Could you check a few things on this model? Use its own coordinates, in mm. Round coordinates to 2 decimals unless told otherwise and drop trailing zeros. Order: outer loops, then holes, each group sorted by start corner. A loop starts at its lowest first (then second) coordinate and runs counter-clockwise, first axis right, second up. Notation, with made-up numbers: (81.25, 80) - (96.25, 80) arc R24 cw to (96.25, 91) - close; hole circle Ø10 at (34.5, 6.25). An arc over 180 degrees is marked (long way). Use one line per item in the form item = value.
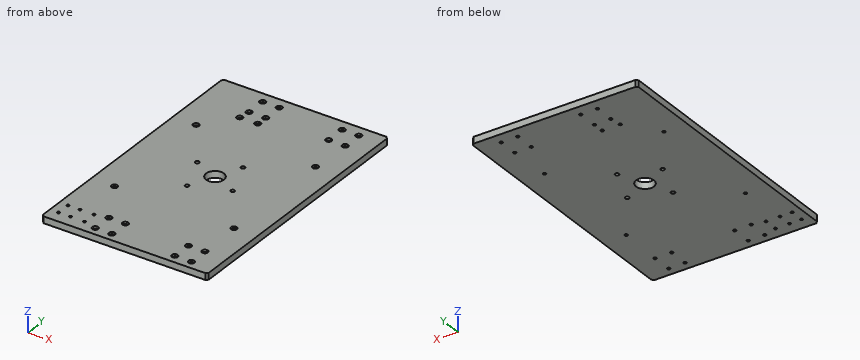
from build123d import *

# Parameters (mm, degrees)
ESQUISSE1_W                                  = 250
ESQUISSE1_H                                  = 400
BOSS_EXTRU_1_DEPTH                           = 10
ESQUISSE2_R                                  = 13.5
ENL_V_MAT_EXTRU_1_DEPTH                      = 237.061432682
CHANFREIN1_SIZE                              = 3
TROU_TARAUD_M51_D                            = 4.2
TROUS_DE_CENTRAGE_4_0MM2_D                   = 4
TROUS_DE_CENTRAGE_6_0MM2_D                   = 6
D_GAGEMENT_M41_D                             = 4.5
R_P_TITION_LIN_AIRE1_COUNT                   = 2
R_P_TITION_LIN_AIRE1_PITCH                   = 120
R_P_TITION_LIN_AIRE1_COUNT_DIR2              = 2
R_P_TITION_LIN_AIRE1_PITCH_DIR2              = 340
R_P_TITION_LIN_AIRE2_COUNT                   = 2
R_P_TITION_LIN_AIRE2_PITCH                   = 30
R_P_TITION_LIN_AIRE2_COUNT_DIR2              = 2
R_P_TITION_LIN_AIRE2_PITCH_DIR2              = 25
R_P_TITION_LIN_AIRE3_COUNT                   = 2
R_P_TITION_LIN_AIRE3_PITCH                   = 120
R_P_TITION_LIN_AIRE3_COUNT_DIR2              = 2
R_P_TITION_LIN_AIRE3_PITCH_DIR2              = 340
D_GAGEMENT_M42_D                             = 4.5
CHAMBRAGE_POUR_VIS_T_TE_RONDE_BOMB_2_A_COUNT = 2
CHAMBRAGE_POUR_VIS_T_TE_RONDE_BOMB_2_A_PITCH = 180
CHAMBRAGE_POUR_VIS_T_TE_RONDE_BOMB_3_COUNT   = 2
CHAMBRAGE_POUR_VIS_T_TE_RONDE_BOMB_3_PITCH   = 180
CHAMBRAGE_POUR_VIS_T_TE_RONDE_BOMB_4_COUNT   = 2
CHAMBRAGE_POUR_VIS_T_TE_RONDE_BOMB_4_PITCH   = 254.558441227
D_GAGEMENT_M43_D                             = 4.5
CHAMBRAGE_POUR_VIS_T_TE_RONDE_BOMB_5_A_COUNT = 2
CHAMBRAGE_POUR_VIS_T_TE_RONDE_BOMB_5_A_PITCH = 26.858717456


with BuildPart() as part:
    # Esquisse1 → Boss.-Extru.1 (new body)
    with BuildSketch(Plane.XY):
        Rectangle(ESQUISSE1_W, ESQUISSE1_H)
    extrude(amount=BOSS_EXTRU_1_DEPTH)

    # Esquisse2 → Enlèv. mat.-Extru.1 (cut, through all)
    with BuildSketch(Plane(origin=(0, 0, 0), x_dir=(-1, 0, 0), z_dir=(0, 0, -1))):
        Circle(ESQUISSE2_R)
    extrude(amount=-ENL_V_MAT_EXTRU_1_DEPTH, mode=Mode.SUBTRACT)

    # Chanfrein1
    chanfrein1_edges = [part.edges().sort_by_distance(p)[0] for p in [
        (125, -200, 5),
        (-125, -200, 5),
        (-125, 200, 5),
        (125, 200, 5),
    ]]
    chamfer(chanfrein1_edges, length=CHANFREIN1_SIZE)

    # Trou taraudé M51 (through all)
    with Locations(Plane.XY.offset(10)):
        with Locations((-72.698486264, -161.07971462), (-72.698486264, -181.838730229), (-111.937151978, -181.838730229), (-111.937151978, -161.07971462)):
            Hole(TROU_TARAUD_M51_D / 2)

    # Trous de centrage Ø4.0mm2 (through all)
    with Locations(Plane.XY.offset(10)):
        with Locations((-93.86308218, -161.07971462), (-93.86308218, -181.838730229)):
            Hole(TROUS_DE_CENTRAGE_4_0MM2_D / 2)

    # Trous de centrage Ø6.0mm2 (through all)
    with Locations(Plane.XY.offset(10)):
        with Locations((16.357059687, 37.86831259), (37.86831259, -16.357059687), (-16.357059687, -37.86831259), (-37.86831259, 16.357059687)):
            Hole(TROUS_DE_CENTRAGE_6_0MM2_D / 2)

    # Dégagement M41 (through all)
    with Locations(Plane(origin=(0, 0, 0), x_dir=(-1, 0, 0), z_dir=(0, 0, -1))):
        with Locations((28, -187), (28, -157), (53, -157), (53, -187)):
            d_gagement_m41 = Hole(D_GAGEMENT_M41_D / 2)

    # Répétition linéaire1: D_gagement M41 2 × 2
    with Locations(*[(i * R_P_TITION_LIN_AIRE1_PITCH, j * R_P_TITION_LIN_AIRE1_PITCH_DIR2, 0) for i in range(R_P_TITION_LIN_AIRE1_COUNT) for j in range(R_P_TITION_LIN_AIRE1_COUNT_DIR2) if (i, j) != (0, 0)]):
        add(d_gagement_m41, mode=Mode.SUBTRACT)

    # Esquisse29 → Chambrage pour vis _ t_te ronde bomb_e M (revolve, cut)
    with BuildSketch(Plane(origin=(92, -157, 10), x_dir=(0, -1, 0), z_dir=(1, 0, 0))):
        Polygon((0, 0), (0, 10), (2.25, 10), (2.25, 3.125), (2.275, 3.1), (4.5, 3.1), (4.5, 0), align=None)
    chambrage_pour_vis_t_te_ronde_bomb_e_m = revolve(axis=Axis((92, -157, 16.35), (0, 0, -1)), mode=Mode.SUBTRACT)

    # Répétition linéaire2: Chambrage pour vis _ t_te ronde bomb_e M 2 × 2
    with Locations(*[(-j * R_P_TITION_LIN_AIRE2_PITCH_DIR2, -i * R_P_TITION_LIN_AIRE2_PITCH, 0) for i in range(R_P_TITION_LIN_AIRE2_COUNT) for j in range(R_P_TITION_LIN_AIRE2_COUNT_DIR2) if (i, j) != (0, 0)]):
        add(chambrage_pour_vis_t_te_ronde_bomb_e_m, mode=Mode.SUBTRACT)

    # Répétition linéaire3: Chambrage pour vis _ t_te ronde bomb_e M 2 × 2
    with Locations(*[(-i * R_P_TITION_LIN_AIRE3_PITCH, j * R_P_TITION_LIN_AIRE3_PITCH_DIR2, 0) for i in range(R_P_TITION_LIN_AIRE3_COUNT) for j in range(R_P_TITION_LIN_AIRE3_COUNT_DIR2) if (i, j) != (0, 0)]):
        add(chambrage_pour_vis_t_te_ronde_bomb_e_m, mode=Mode.SUBTRACT)

    # Répétition linéaire3 copy 1 sketch → Répétition linéaire3 copy 1 (revolve, cut)
    with BuildSketch(Plane(origin=(67, 183, 10), x_dir=(0, -1, 0), z_dir=(1, 0, 0))):
        Polygon((0, 0), (0, 10), (2.25, 10), (2.25, 3.125), (2.275, 3.1), (4.5, 3.1), (4.5, 0), align=None)
    revolve(axis=Axis((67, 183, 16.35), (0, 0, -1)), mode=Mode.SUBTRACT)

    # Répétition linéaire3 copy 2 sketch → Répétition linéaire3 copy 2 (revolve, cut)
    with BuildSketch(Plane(origin=(-53, -157, 10), x_dir=(0, -1, 0), z_dir=(1, 0, 0))):
        Polygon((0, 0), (0, 10), (2.25, 10), (2.25, 3.125), (2.275, 3.1), (4.5, 3.1), (4.5, 0), align=None)
    revolve(axis=Axis((-53, -157, 16.35), (0, 0, -1)), mode=Mode.SUBTRACT)

    # Répétition linéaire3 copy 3 sketch → Répétition linéaire3 copy 3 (revolve, cut)
    with BuildSketch(Plane(origin=(-53, 183, 10), x_dir=(0, -1, 0), z_dir=(1, 0, 0))):
        Polygon((0, 0), (0, 10), (2.25, 10), (2.25, 3.125), (2.275, 3.1), (4.5, 3.1), (4.5, 0), align=None)
    revolve(axis=Axis((-53, 183, 16.35), (0, 0, -1)), mode=Mode.SUBTRACT)

    # Répétition linéaire3 copy 4 sketch → Répétition linéaire3 copy 4 (revolve, cut)
    with BuildSketch(Plane(origin=(92, 153, 10), x_dir=(0, -1, 0), z_dir=(1, 0, 0))):
        Polygon((0, 0), (0, 10), (2.25, 10), (2.25, 3.125), (2.275, 3.1), (4.5, 3.1), (4.5, 0), align=None)
    revolve(axis=Axis((92, 153, 16.35), (0, 0, -1)), mode=Mode.SUBTRACT)

    # Répétition linéaire3 copy 5 sketch → Répétition linéaire3 copy 5 (revolve, cut)
    with BuildSketch(Plane(origin=(-28, -187, 10), x_dir=(0, -1, 0), z_dir=(1, 0, 0))):
        Polygon((0, 0), (0, 10), (2.25, 10), (2.25, 3.125), (2.275, 3.1), (4.5, 3.1), (4.5, 0), align=None)
    revolve(axis=Axis((-28, -187, 16.35), (0, 0, -1)), mode=Mode.SUBTRACT)

    # Répétition linéaire3 copy 6 sketch → Répétition linéaire3 copy 6 (revolve, cut)
    with BuildSketch(Plane(origin=(-28, 153, 10), x_dir=(0, -1, 0), z_dir=(1, 0, 0))):
        Polygon((0, 0), (0, 10), (2.25, 10), (2.25, 3.125), (2.275, 3.1), (4.5, 3.1), (4.5, 0), align=None)
    revolve(axis=Axis((-28, 153, 16.35), (0, 0, -1)), mode=Mode.SUBTRACT)

    # Répétition linéaire3 copy 7 sketch → Répétition linéaire3 copy 7 (revolve, cut)
    with BuildSketch(Plane(origin=(67, 153, 10), x_dir=(0, -1, 0), z_dir=(1, 0, 0))):
        Polygon((0, 0), (0, 10), (2.25, 10), (2.25, 3.125), (2.275, 3.1), (4.5, 3.1), (4.5, 0), align=None)
    revolve(axis=Axis((67, 153, 16.35), (0, 0, -1)), mode=Mode.SUBTRACT)

    # Répétition linéaire3 copy 8 sketch → Répétition linéaire3 copy 8 (revolve, cut)
    with BuildSketch(Plane(origin=(-53, -187, 10), x_dir=(0, -1, 0), z_dir=(1, 0, 0))):
        Polygon((0, 0), (0, 10), (2.25, 10), (2.25, 3.125), (2.275, 3.1), (4.5, 3.1), (4.5, 0), align=None)
    revolve(axis=Axis((-53, -187, 16.35), (0, 0, -1)), mode=Mode.SUBTRACT)

    # Répétition linéaire3 copy 9 sketch → Répétition linéaire3 copy 9 (revolve, cut)
    with BuildSketch(Plane(origin=(-53, 153, 10), x_dir=(0, -1, 0), z_dir=(1, 0, 0))):
        Polygon((0, 0), (0, 10), (2.25, 10), (2.25, 3.125), (2.275, 3.1), (4.5, 3.1), (4.5, 0), align=None)
    revolve(axis=Axis((-53, 153, 16.35), (0, 0, -1)), mode=Mode.SUBTRACT)

    # Dégagement M42 (through all)
    with Locations(Plane(origin=(0, 0, 0), x_dir=(-1, 0, 0), z_dir=(0, 0, -1))):
        with Locations((90, -90), (90, 90), (-90, 90), (-90, -90)):
            Hole(D_GAGEMENT_M42_D / 2)

    # Esquisse33 → Chambrage pour vis _ t_te ronde bomb 2 (revolve, cut)
    with BuildSketch(Plane(origin=(-90, -90, 10), x_dir=(0, -1, 0), z_dir=(1, 0, 0))):
        Polygon((0, 0), (0, 10), (2.25, 10), (2.25, 3.125), (2.275, 3.1), (4.5, 3.1), (4.5, 0), align=None)
    chambrage_pour_vis_t_te_ronde_bomb_2 = revolve(axis=Axis((-90, -90, 16.35), (0, 0, -1)), mode=Mode.SUBTRACT)

    # Chambrage pour vis _ t_te ronde bomb 2 a: Chambrage pour vis _ t_te ronde bomb 2 ×2
    with Locations(*[(0, i * CHAMBRAGE_POUR_VIS_T_TE_RONDE_BOMB_2_A_PITCH, 0) for i in range(1, CHAMBRAGE_POUR_VIS_T_TE_RONDE_BOMB_2_A_COUNT)]):
        add(chambrage_pour_vis_t_te_ronde_bomb_2, mode=Mode.SUBTRACT)

    # Chambrage pour vis _ t_te ronde bomb 3: Chambrage pour vis _ t_te ronde bomb 2 ×2
    with Locations(*[(i * CHAMBRAGE_POUR_VIS_T_TE_RONDE_BOMB_3_PITCH, 0, 0) for i in range(1, CHAMBRAGE_POUR_VIS_T_TE_RONDE_BOMB_3_COUNT)]):
        add(chambrage_pour_vis_t_te_ronde_bomb_2, mode=Mode.SUBTRACT)

    # Chambrage pour vis _ t_te ronde bomb 4: Chambrage pour vis _ t_te ronde bomb 2 ×2
    with Locations(*[Vector(0.7071067811864814, 0.7071067811866137, 0) * (i * CHAMBRAGE_POUR_VIS_T_TE_RONDE_BOMB_4_PITCH) for i in range(1, CHAMBRAGE_POUR_VIS_T_TE_RONDE_BOMB_4_COUNT)]):
        add(chambrage_pour_vis_t_te_ronde_bomb_2, mode=Mode.SUBTRACT)

    # Dégagement M43 (through all)
    with Locations(Plane(origin=(0, 0, 0), x_dir=(-1, 0, 0), z_dir=(0, 0, -1))):
        with Locations((55.199022773, 135.70653433), (28.341819814, 135.991758108)):
            Hole(D_GAGEMENT_M43_D / 2)

    # Esquisse37 → Chambrage pour vis _ t_te ronde bomb 5 (revolve, cut)
    with BuildSketch(Plane(origin=(-55.199022773, 135.70653433, 10), x_dir=(0, -1, 0), z_dir=(1, 0, 0))):
        Polygon((0, 0), (0, 10), (2.25, 10), (2.25, 3.125), (2.275, 3.1), (4.5, 3.1), (4.5, 0), align=None)
    chambrage_pour_vis_t_te_ronde_bomb_5 = revolve(axis=Axis((-55.199022773, 135.70653433, 16.35), (0, 0, -1)), mode=Mode.SUBTRACT)

    # Chambrage pour vis _ t_te ronde bomb 5 a: Chambrage pour vis _ t_te ronde bomb 5 ×2
    with Locations(*[Vector(0.9999436124580966, 0.010619411671655749, 0) * (i * CHAMBRAGE_POUR_VIS_T_TE_RONDE_BOMB_5_A_PITCH) for i in range(1, CHAMBRAGE_POUR_VIS_T_TE_RONDE_BOMB_5_A_COUNT)]):
        add(chambrage_pour_vis_t_te_ronde_bomb_5, mode=Mode.SUBTRACT)


solid = part.part
Item 1: Imagine slicing it at A-A on y = 0. Please give me the cut outline in (x, z), plus the area to 3 significant figures.
Found:
outline = (-125, 0) - (-13.5, 0) - (-13.5, 10) - (-125, 10) - close; (13.5, 0) - (125, 0) - (125, 10) - (13.5, 10) - close
area = 2,230 mm2
Item 2: Imagine slicing it at B-B on x = -6. Please give me the cut outline in (y, z).
Found:
outline = (-200, 0) - (-12.09, 0) - (-12.09, 10) - (-200, 10) - close; (12.09, 0) - (200, 0) - (200, 10) - (12.09, 10) - close
Item 3: I need wall thicknesses on L1, parallel to X at y = -187, z = 4.25; L2, parallel to Y at x = -28, z = 7.7; L3, parallel to X at y = 183, z = 8.75. Which ranges of each line are inside material? Lowest first, please.
Found:
L1 = -125 to -55.25, -50.75 to -30.25, -25.75 to 64.75, 69.25 to 89.75, 94.25 to 125
L2 = -200 to -191.5, -182.5 to -161.5, -152.5 to 131.5, 140.48 to 148.5, 157.5 to 178.5, 187.5 to 200
L3 = -125 to -57.5, -48.5 to -32.5, -23.5 to 62.5, 71.5 to 87.5, 96.5 to 125
Item 4: Will this pin go through, and if not, where does the flat tip stop? P1, Ø4.5, axis at x = 65.5, y = -185.5, coming from the +Z side.
Found:
P1 = 6.9
